Autodesk Inventor part; units mm, degrees
ref_plane "YZ Plane" through (0, 0, 0) normal (1, 0, 0) x (0, 1, 0)
ref_plane "XZ Plane" through (0, 0, 0) normal (0, 1, 0) x (-1, 0, 0)
ref_plane "XY Plane" through (0, 0, 0) normal (0, 0, 1) x (1, 0, 0)
sketch "Sketch1" plane through (0, 0, 0) normal (0, 1, 0) x (-1, 0, 0)
  line L0 (-2, 0) -> (2, 0)
  line L1 (2, 0) -> (2, 12.1)
  line L2 (2, 12.1) -> (-2, 12.1)
  line L3 (-2, 12.1) -> (-2, 0)
  point P0 (0, 0)
  point P1 (0, 0)
  dimension "d0" = 4
  dimension "d1" = 12.1
extrude "Extrusion1" add sketch "Sketch1" along normal mid plane 2
chamfer "Chamfer1" distance 1.4 distance2 0.45 1 edges at (-2, 0, 12.1) measured on face at (-2, 0.3333, 8.0667)
chamfer "Chamfer2" distance 1.4 distance2 0.45 1 edges at (2, 0, 12.1) measured on face at (2, -0.3333, 8.0667)
chamfer "Chamfer3" distance 1.4 distance2 0.75 1 edges at (0, 1, 12.1) measured on face at (0.6667, 1, 7.1333)
chamfer "Chamfer4" distance 1.4 distance2 0.75 1 edges at (0, -1, 12.1) measured on face at (0.6667, -1, 7.1333)
properties material "Nickel-Copper Alloy 400"
For this review, take the finished solid that the model builds, in its own axes (mm). Coordinates: 2 decimals unless noted, no trailing zeros. Loops run counter-clockwise (first coordinate to the right, second up) from the corner with the lowest first, then second, coordinate; pieces in that order, holes last. Notation, with made-up numbers: (-32, -17.75) -> (27, -17.75) arc R4 cw to (27, -12.75) -> close; hole circle Ø2 at (46.25, -33.5). An arc over 180 degrees is marked (long way). Write each question's results on one line, items separated by ' | '.
Q1. Add section B-B, the plane y = 0.7. State the section outline as (x, z) points, then the cut area to 3 significant figures.
Taken from the geometry:
outline: (-2, 0) -> (2, 0) -> (2, 10.7) -> (1.82, 11.26) -> (-1.82, 11.26) -> (-2, 10.7) -> close | area: 44.9 mm²
Q2. For pin 1 Ø1 at (x, y) = (-0.5, 0) entering from -Z, flat-tipped, find the tip position at first contact; note if it passes through.
Taken from the geometry:
pin 1: z = 0
Q3. To check wall thickness, follow line 1 along Z through (x, y) = (1.05, 0.6); line 2 along Z through (x, y) = (0.2, -0.3); line 3 along Y through (x, z) = (1.5, 11.5). State the ranges of each line that lie inside material, in increasing order. Write a range as [from, to].
Taken from the geometry:
line 1: [0, 11.45] | line 2: [0, 12.01] | line 3: [-0.57, 0.57]
Q4. Add section A-A, the plane x = -1.4. State the section outline as (y, z) points, then the cut area to 4 significant figures.
Taken from the geometry:
outline: (-1, 0) -> (1, 0) -> (1, 10.7) -> (0.25, 12.1) -> (-0.25, 12.1) -> (-1, 10.7) -> close | area: 23.15 mm²
